Autodesk Inventor part; units mm, degrees
ref_plane "Work Plane1" through (99.4266, 0, -12.9365) normal (0.9848078, -0.1736482, 0) x (0, 0, -1)
ref_plane "Work Plane2" through (-102.6005, 6, 0) normal (0, 0, 1) x (1, 0, 0)
ref_plane "Work Plane3" through (-101.5425, 12, -61.3094) normal (0.1735668, -0.0306045, -0.9843464) x (0.9848078, 0, 0.1736482)
sketch "Sketch1" plane through (0, 0, 0) normal (0, 1, 0) x (-1, 0, 0)
  line L0 (101.5425, -61.3094) -> (101.5425, 0)
  line L1 (101.5425, 0) -> (-101.5425, 0)
  line L2 (-101.5425, 0) -> (-101.5425, -25.5)
  line L3 (-101.5425, -25.5) -> (101.5425, -61.3094)
  point P0 (0, 0)
  point P1 (0, 0)
  dimension "d0" = 100
  dimension "d1" = 25.5
  dimension "d5" = 203.085
  dimension "d15" = 25.5
  dimension "d16" = 156.1695
extrude "Extrusion1" add sketch "Sketch1" along normal blind 12
draft "FaceDraft2" angle 10 pull direction (0, -1, 0) faces at (101.5425, 4, -8.5) fixed edges at (101.5425, 12, -12.75)
draft "FaceDraft3" angle -10 pull direction (0, -1, 0) faces at (-101.5425, 4, -40.8729) fixed edges at (-101.5425, 12, -30.6547)
properties part number "Panel_side"
Build history of the part. All positions in model axes, mm. Round coordinates to 2 decimals unless told otherwise and drop trailing zeros. Write each loop counter-clockwise with the first axis right and the second up, starting at its lowest first coordinate (ties: lowest second). Pieces come first, ordered by that corner, then holes.
1) Drill centre lines: probe 1 along Z at (x, y) = (-39, 10.75); probe 2 along Z at (x, y) = (-56, 11.5); probe 3 along X at (y, z) = (3.5, -12). Where is each one in solid material? Low to high.
2) Pin check, flat tips, straight feed: pin 1 (1.5 mm diameter, centred on y = 8.5, z = -11.5, fed in from +X); pin 2 (1.5 mm diameter, centred on y = 4, z = -53.5, fed in from -X); pin 3 (4 mm diameter, centred on y = 9, z = -27, fed in from +X). Stop position of each tip, or through.
3) Band-saw the part on B-B, the plane y = 6.75. List the corners of the cut face in (x, z), and give its area (3 significant figures).
4) Band-saw the part on A-A, the plane z = -44. List the corners of the cut face in (x, y), and give its area (3 significant figures).
5) Mould opens along X. For faces 1 (the flat face through (-23, 0, -24)), 2 (the flat face through (100.47, 5.92, -12.76)), 3 (the flat face through (-102.615, 5.916, -31.273)) say: +X half, -X half, draft (parallel to the pull), parting line (faces both ways), or undercut.
Ans:
1. probe 1: z = -50.28 to 0
1. probe 2: z = -53.28 to 0
1. probe 3: x = -103.04 to 100.04
2. pin 1: stops at x = 101.06
2. pin 2: stops at x = -103.09
2. pin 3: stops at x = 101.26
3. outline: (-102.47, -61.47) - (100.62, -25.66) - (100.62, 0) - (-102.47, 0) - close
3. area: 8,850 mm2
4. outline: (-103.66, 0) - (-3.38, 0) - (-3.38, 12) - (-101.54, 12) - close
4. area: 1,190 mm2
5. face 1: draft
5. face 2: +X half
5. face 3: -X half
